Study the drawing (mm; zero at the part's minimum x, y, z) and answer. A direction names the side the tool comes from. Coordinates: 2 decimals unless noted, no trailing zeros. Order: outer loops, then holes, each group sorted by start corner. A loop starts at its lowest first (then second) coordinate and runs counter-clockwise, first axis right, second up. Notation, with made-up numbers: M -33.75,71 L -10.75,71 A21 cw -10.75,75 Z; hole C 53.25,23 d10. An arc over 180 degrees is marked long. Use a Markdown table: item, result. Add a question column.
1) Find section A-A on y = 5.25. Write down the section's boundary in (x, z), plus the area to 3 significant figures.
2) Find the intervals of material crossed by probe 1 along Y at (x, z) = (18, 7.5); probe 2 along Z at (x, y) = (13.5, 6); probe 3 along Y at (x, z) = (10, 11.25), in increasing order. Write a range as [from, to].
3) For the marked faces 1 and 2, determine the directions among +Z, -Z, +X, -X, +Y, -Y from which every point of the face is accessible in a straight line to the end or side of a thin tool.
4) Each of these flat-tipped pins is pushed along its axis until it touches: pin 1 Ø1.5 at (x, y) = (11, 11) entering from +Z; pin 2 Ø4 at (y, z) = (16, 11) entering from -X; pin 3 Ø2 at (x, y) = (8.5, 15) entering from -Z. Where does it stop, or does it pass through?
5) Find section B-B on y = 17.75. Write down the section's boundary in (x, z) (3 decimals), plus the area to 3 significant figures.
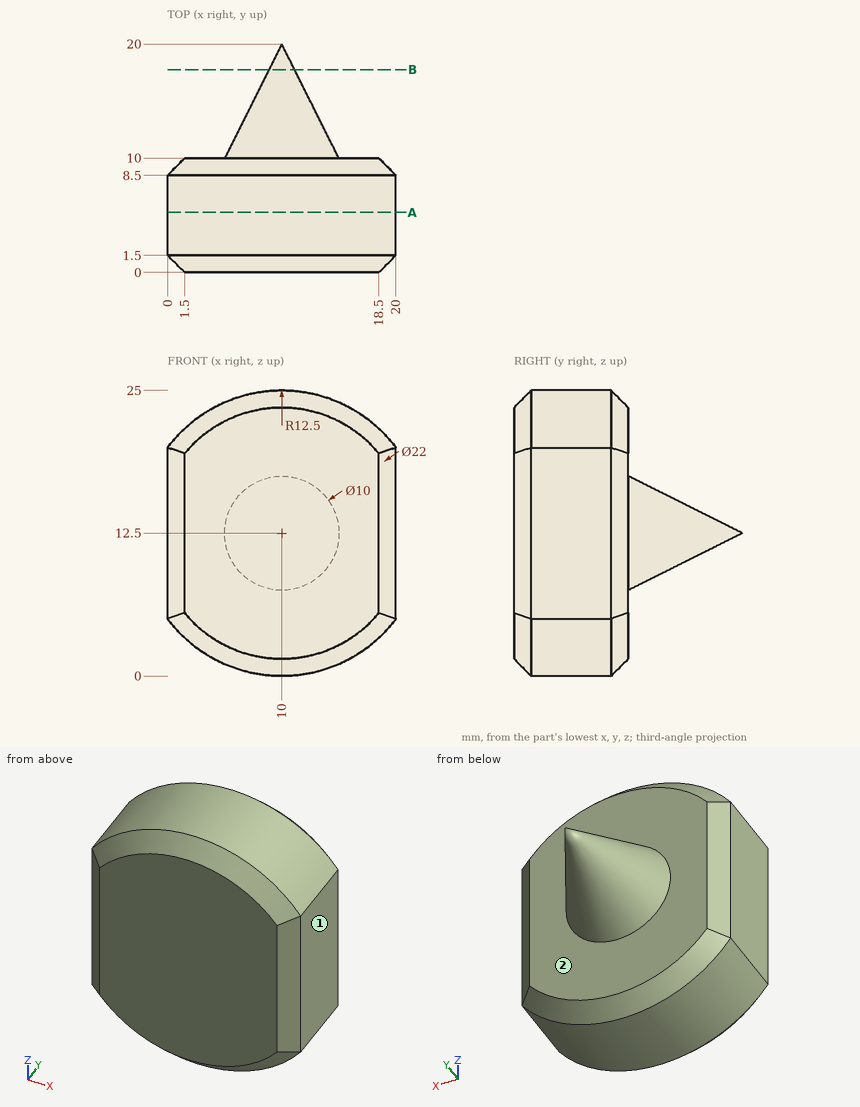
Check result:
| question | item | result |
|---|---|---|
| 1 | outline | M 0,5 A12.5 ccw 20,5 L 20,20 A12.5 ccw 0,20 Z |
| 1 | area | 440 mm2 |
| 2 | probe 1 | y = [0, 10] |
| 2 | probe 2 | z = [0.5, 24.5] |
| 2 | probe 3 | y = [0, 17.5] |
| 3 | face 1 | +Z, -Z, +X, +Y, -Y |
| 3 | face 2 | +Y |
| 4 | pin 1 | stops at z = 17.3 |
| 4 | pin 2 | stops at x = 7.17 |
| 4 | pin 3 | stops at z = 9.74 |
| 5 | outline | C 10,12.5 d2.25 |
| 5 | area | 3.98 mm2 |
